from build123d import *

# Parameters (mm, degrees)
SKETCH_W        = 44
SKETCH_H        = 15
SKETCH_R        = 1.7
PAD_DEPTH       = 2
CHAMFER_SIZE    = 1.5
SKETCH001_W     = 2
SKETCH001_H     = 15
SKETCH001_W_2   = 6
PAD001_DEPTH    = 8
FILLET_R        = 4.5
SKETCH002_R     = 1.5
POCKET_DEPTH    = 8
CHAMFER001_SIZE = 5.5
FILLET001_R     = 4
CHAMFER002_SIZE = 1


with BuildPart() as part:
    # Sketch → Pad (new body)
    with BuildSketch(Plane.XY):
        with Locations((22, 7.5)):
            Rectangle(SKETCH_W, SKETCH_H)
        with Locations((4, 7.5)):
            Circle(SKETCH_R, mode=Mode.SUBTRACT)
        with Locations((40, 7.5)):
            Circle(SKETCH_R, mode=Mode.SUBTRACT)
    extrude(amount=PAD_DEPTH)

    # Chamfer
    chamfer_edges = [part.edges().sort_by_distance(p)[0] for p in [
        (2.3, 7.5, 2),
        (38.3, 7.5, 2),
    ]]
    chamfer(chamfer_edges, length=CHAMFER_SIZE)

    # Sketch001 (on Face4 of Chamfer) → Pad001 (join)
    with BuildSketch(Plane.XY.offset(2)):
        with Locations((8.5, 7.5)):
            Rectangle(SKETCH001_W, SKETCH001_H)
        with Locations((35.5, 7.5)):
            Rectangle(SKETCH001_W, SKETCH001_H)
        with Locations((22, 7.5)):
            Rectangle(SKETCH001_W_2, SKETCH001_H)
    extrude(amount=PAD001_DEPTH)

    # Fillet
    fillet_edges = [part.edges().sort_by_distance(p)[0] for p in [
        (9.5, 7.5, 2),
        (19, 7.5, 2),
        (25, 7.5, 2),
        (34.5, 7.5, 2),
    ]]
    fillet(fillet_edges, radius=FILLET_R)

    # Sketch002 (on Face20 of Fillet) → Pocket (cut)
    with BuildSketch(Plane.XY.offset(10)):
        with Locations((22, 7.5)):
            Circle(SKETCH002_R)
    extrude(amount=-POCKET_DEPTH, mode=Mode.SUBTRACT)

    # Chamfer001
    chamfer001_edges = [part.edges().sort_by_distance(p)[0] for p in [
        (0, 0, 1),
        (0, 15, 1),
        (44, 15, 1),
        (44, 0, 1),
    ]]
    chamfer(chamfer001_edges, length=CHAMFER001_SIZE)

    # Fillet001
    fillet001_edges = [part.edges().sort_by_distance(p)[0] for p in [
        (0, 5.5, 1),
        (0, 9.5, 1),
        (44, 9.5, 1),
        (44, 5.5, 1),
    ]]
    fillet(fillet001_edges, radius=FILLET001_R)

    # Chamfer002
    chamfer002_edges = [part.edges().sort_by_distance(p)[0] for p in [
        (20.5, 7.5, 10),
    ]]
    chamfer(chamfer002_edges, length=CHAMFER002_SIZE)


solid = part.part
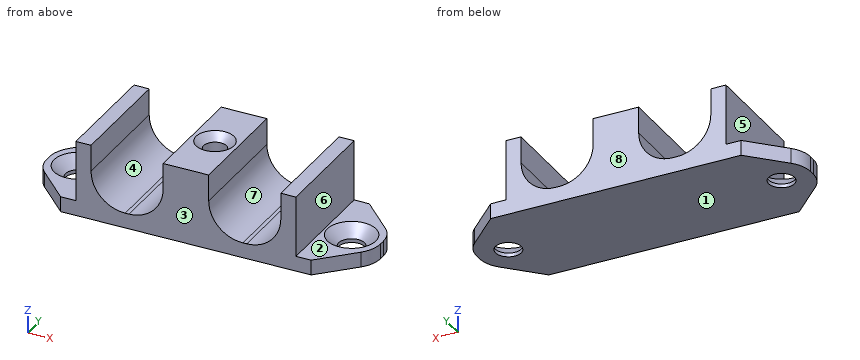
Here's how the part is built. I have some questions about the finished solid (model axes, mm). Face numbers are marked on the shaded views. A direction names the side the tool comes from. Coordinates: 2 decimals unless noted, no trailing zeros. Order: outer loops, then holes, each group sorted by start corner. A loop starts at its lowest first (then second) coordinate and runs counter-clockwise, first axis right, second up. Notation, with made-up numbers: (31.25, 35.25) - (51.25, 35.25) arc R18 cw to (51.25, 59.25) - close; hole circle Ø11 at (30, 49). An arc over 180 degrees is marked (long way). Use CSV: the item, a comma, the result in double quotes. Start each with the question number.
1. Please list where these lines run through material, in increasing order: line 1 (Y direction, x = 22, z = 6.75); line 2 (X direction, y = 1, z = 3); line 3 (X direction, y = 13.5, z = 7). Write a range as from..to.
2. Suppose I cut it at A-A on z = 4.25. List the corners of the cut face in (x, y) for me.
3. I'm going to push flat-ended pins straight in: pin 1 (4 mm diameter, centred on y = 8.5, z = 8.5, fed in from -X); pin 2 (2.5 mm diameter, centred on x = 22, y = 7.5, fed in from +Z); pin 3 (6 mm diameter, centred on y = 12.5, z = 7, fed in from +X). Where does each tip first touch, or does it pass through?
4. For the marked faces 1, 2, 3, 4 and 5, which set-ups out of +Z, -Z, +X, -X, +Y, -Y let a thin tool reach every point of the face, with its end or its side?
5. Suppose I cut it at B-B on x = 4. List the corners of the cut face in (y, z) for me.
6. If we mould it in two halves opening along X, with no side actions, what happens to the marked faces 6, 7 and 8? For each: +X half, -X half, draft (parallel to the pull), parting line (faces both ways), or undercut.
7. Suppose I cut it at D-D on x = 22. List the corners of the cut face in (y, z) for me.
8. Suppose I cut it at C-C on y = 2. List the corners of the cut face in (x, z) for me, then the cut area to 3 significant figures.
Output:
1,line 1,"y = 0..6, 9..15"
1,line 2,"x = 7.5..11.17, 17.33..26.67, 32.83..36.5"
1,line 3,"x = 7.5..9.5, 19..25, 34.5..36.5"
2,outline,"(7.5, 0) - (10.1, 0) - (10.1, 15) - (7.5, 15) - close; (18.4, 0) - (25.6, 0) - (25.6, 15) - (18.4, 15) - close; (33.9, 0) - (36.5, 0) - (36.5, 15) - (33.9, 15) - close; hole circle Ø3 at (22, 7.5)"
3,pin 1,"stops at x = 7.5"
3,pin 2,"stops at z = 2"
3,pin 3,"stops at x = 36.5"
4,face 1,"-Z, +X, -X, +Y, -Y"
4,face 2,"+Z, +X, +Y, -Y"
4,face 3,"+Z, -Z, +X, -X, -Y"
4,face 4,"+Z, +Y, -Y"
4,face 5,"+Z, -X, +Y, -Y"
5,outline,"(1.5, 0) - (5.8, 0) - (5.8, 0.5) - (4.3, 2) - (1.5, 2) - close; (9.2, 0) - (13.5, 0) - (13.5, 2) - (10.7, 2) - (9.2, 0.5) - close"
6,face 6,"+X half"
6,face 7,"undercut"
6,face 8,"draft"
7,outline,"(0, 0) - (15, 0) - (15, 10) - (10, 10) - (9, 9) - (9, 2) - (6, 2) - (6, 9) - (5, 10) - (0, 10) - close"
8,outline,"(3.5, 0) - (40.5, 0) - (40.5, 2) - (36.5, 2) - (36.5, 10) - (34.5, 10) - (34.5, 6.5) arc R4.5 cw to (30, 2) - (29.5, 2) arc R4.5 cw to (25, 6.5) - (25, 10) - (19, 10) - (19, 6.5) arc R4.5 cw to (14.5, 2) - (14, 2) arc R4.5 cw to (9.5, 6.5) - (9.5, 10) - (7.5, 10) - (7.5, 2) - (3.5, 2) - close"
8,area,"171 mm2"
